Autodesk Inventor part; units mm, degrees
ref_plane "YZ Plane" through (0, 0, 0) normal (1, 0, 0) x (0, 1, 0)
ref_plane "XZ Plane" through (0, 0, 0) normal (0, 1, 0) x (-1, 0, 0)
ref_plane "XY Plane" through (0, 0, 0) normal (0, 0, 1) x (1, 0, 0)
sketch "Sketch1" plane through (0, 0, 0) normal (0, 0, 1) x (1, 0, 0)
  line L0 (10, -10) -> (-10, -10)
  line L1 (-10, -10) -> (-10, 10)
  line L2 (-10, 10) -> (10, 10)
  line L3 (10, 10) -> (10, -10)
  circle A0 centre (0, 5) radius 1.2
  circle A1 centre (0, -5) radius 1.2
  circle A2 centre (0, 0) radius 3
  dimension "d0" = 10
  dimension "d1" = 10
  dimension "d2" = 10
  dimension "d3" = 10
  dimension "d4" = 5
  dimension "d5" = 5
  dimension "d6" = 2.4
  dimension "d7" = 2.4
  dimension "d8" = 6
extrude "Extrusion1" add sketch "Sketch1" along normal blind 4
sketch "Sketch2" plane through (0, 0, 4) normal (0, 0, 1) x (1, 0, 0)
  line L0 (0, 0) -> (-1.3346, -1.3533)
  line L1 (10, 10) -> (-10, 10)
  line L2 (10, -9.9996) -> (6, -9.9996)
  line L3 (6, -9.9996) -> (6, 10)
  line L4 (6, 10) -> (10, 10)
  line L5 (10, 10) -> (10, -9.9996)
  line L6 (8, -1.9998) -> (4, -1.9998)
  line L7 (4, -1.9998) -> (4, 2.0002)
  line L8 (4, 2.0002) -> (8, 2.0002)
  line L9 (8, 2.0002) -> (8, -1.9998)
  line L10 (8, -1.9998) -> (4, 2.0002) construction
  line L11 (4, -1.9998) -> (8, 2.0002) construction
  point P0 (6, 0.0002)
  point P1 (6, -1.9998)
  point P2 (6, 2.0002)
  dimension "d19" = 6
  dimension "d20" = 10
  dimension "d21" = 4
  dimension "d22" = 4
extrude "Extrusion2" add sketch "Sketch2" along normal blind 40
sketch "Sketch3" plane through (0, 0, 44) normal (0, 0, 1) x (1, 0, 0)
  line L0 (10, 10) -> (-10, 10)
  line L1 (10, -10) -> (-10, -10)
  line L2 (-10, -10) -> (-10, 10)
  line L3 (-10, 10) -> (10, 10)
  line L4 (10, 10) -> (10, -10)
  line L5 (10, -10) -> (-10, 10) construction
  line L6 (-10, -10) -> (10, 10) construction
  point P0 (0, 0)
extrude "Extrusion3" add sketch "Sketch3" along normal blind 4
equation "\"d7\" = d6"
properties part number "MotorMount"
Here's how the part is built. I have some questions about the finished solid (model axes, mm). A direction names the side the tool comes from. Coordinates: 2 decimals unless noted, no trailing zeros. Order: outer loops, then holes, each group sorted by start corner. A loop starts at its lowest first (then second) coordinate and runs counter-clockwise, first axis right, second up. Notation, with made-up numbers: M -17,75 L 20,75 A5 cw 20,81 Z; hole C 68.5,2 d10. An arc over 180 degrees is marked long. Answer as a JSON object with one key per item and string values. Group by question number.
(1) Suppose I cut it at A-A, the plane x = 0. Please give me the cut outline in (y, z).
(2) Suppose I cut it at D-D, the plane z = 15.5. Please give me the cut outline in (x, y), then the cut area to 3 significant figures.
(3) Suppose I cut it at B-B, the plane y = 5. Please give me the cut outline in (x, z).
(4) I need wall thicknesses on probe 1 along Y at (x, z) = (0, 1.5); probe 2 along Z at (x, y) = (2.25, 8.75); probe 3 along X at (y, z) = (1.25, 23.5). Which ranges of each line are inside material? Lowest first, please.
(5) Suppose I cut it at C-C, the plane x = -8.5. Please give me the cut outline in (y, z), then the cut area to 3 significant figures.
(6) If we mould it in two halves opening along X, with no side actions, what happens to faces 1 (the face through (0.65, -6.01, 1.97)), 2 (the face through (6, 6, 24)), 3 (the face through (-2.4, 2.4, 0))? For each: released by +X, released by -X, zero draft, split by the parting line, or undercut.
(7) For pin 1 (9 mm diameter, centred on y = -6, z = 17, fed in from -X); pin 2 (1.9 mm diameter, centred on x = 0, y = -5, fed in from -Z); pin 3 (4 mm diameter, centred on y = 5, z = 21, fed in from -X); pin 4 (1.5 mm diameter, centred on x = 4.5, y = -5.5, fed in from -Z), each with a flat end and sliding along its axis, tell me the tip position at first contact or that it passes through.
(8) Which directions (+Z, -Z, +X, -X, +Y, -Y) give clear straight access to the entire face, cutting with the end or side of a thin tool? Please do faces 4 (the face through (4, 0, 24)), 5 (the face through (5, 2, 24)), 6 (the face through (-3, 0, 2)), 7 (the face through (6, -6, 24)).
Values found:
{
 "1": {"outline": "M -10,0 L -6.2,0 L -6.2,4 L -10,4 Z; M -10,44 L 10,44 L 10,48 L -10,48 Z; M -3.8,0 L -3,0 L -3,4 L -3.8,4 Z; M 3,0 L 3.8,0 L 3.8,4 L 3,4 Z; M 6.2,0 L 10,0 L 10,4 L 6.2,4 Z"},
 "2": {"outline": "M 4,-2 L 6,-2 L 6,-10 L 10,-10 L 10,10 L 6,10 L 6,2 L 4,2 Z", "area": "88.0 mm^2"},
 "3": {"outline": "M -10,0 L -1.2,0 L -1.2,4 L -10,4 Z; M -10,44 L 6,44 L 6,4 L 1.2,4 L 1.2,0 L 10,0 L 10,48 L -10,48 Z"},
 "4": {"probe 1": "y = -10 to -6.2, -3.8 to -3, 3 to 3.8, 6.2 to 10", "probe 2": "z = 0 to 4, 44 to 48", "probe 3": "x = 4 to 10"},
 "5": {"outline": "M -10,0 L 10,0 L 10,4 L -10,4 Z; M -10,44 L 10,44 L 10,48 L -10,48 Z", "area": "160 mm^2"},
 "6": {"face 1": "undercut", "face 2": "released by -X", "face 3": "zero draft"},
 "7": {"pin 1": "stops at x = 4", "pin 2": "stops at z = 44", "pin 3": "stops at x = 6", "pin 4": "stops at z = 0"},
 "8": {"face 4": "-X, +Y, -Y", "face 5": "-X, +Y", "face 6": "-Z", "face 7": "-X, -Y"}
}
